Verification items for the finished model (mm, model axes). A direction names the side the tool comes from. Give positions to 0.01 mm unless a question says otherwise; leave off trailing zeros. Loops run counter-clockwise (first coordinate to the right, second up) from the corner with the lowest first, then second, coordinate; pieces in that order, holes last. Notation, with made-up numbers: M 24.5,71.25 L 68.5,71.25 A13 ccw 68.5,84.25 Z; hole C -4.5,58 d1. An arc over 180 degrees is marked long. Put each result on its own line as item: value. Start each with the question number.
from build123d import *

# Parameters (mm, degrees)
BOSS_EXTRUDE1_DEPTH = 79.7052
SKETCH5_R           = 5.499261314
SKETCH5_R_2         = 4.7625
CUT_EXTRUDE2_DEPTH  = 7.9375


with BuildPart() as part:
    # Sketch1 → Boss-Extrude1 (new body)
    with BuildSketch(Plane.XY):
        Polygon((2.806881074, 4.728984419), (-2.691980104, 4.795322525), (-5.498861178, 0.066338106), (-2.806881074, -4.728984419), (2.691980104, -4.795322525), (5.498861178, -0.066338106), align=None)
    extrude(amount=BOSS_EXTRUDE1_DEPTH)

    # Sketch5 → Cut-Extrude2 (cut)
    with BuildSketch(Plane.XY.offset(79.7052)):
        Circle(SKETCH5_R)
        Circle(SKETCH5_R_2, mode=Mode.SUBTRACT)
    extrude(amount=-CUT_EXTRUDE2_DEPTH, mode=Mode.SUBTRACT)


solid = part.part
Q1. Scan lines: L1, parallel to Y at x = -1.5, z = 31; L2, parallel to Y at x = 0.5, z = 4; L3, parallel to Z at x = 2.75, y = 4. Record each from-to range of solid material in increasing order.
Q2. Cross-section at A-A, the plane z = 15. Record the boundary of the cut face in (x, y).
Q3. Set-up check for faces 1 (the face through (-3.78, -2.9, 75.79)), 2 (the face through (-2.4, -4.3, 71.768)), 3 (the face through (2.5, -4.3, 71.768)), 4 (the face through (-2.34, 4.32, 71.768)): record each of +Z, -Z, +X, -X, +Y, -Y from which the full face is reachable in a straight line by a thin tool's end or side.
Q4. Go/stop test with flat-tipped pins: pin 1 (1 mm diameter, centred on x = -0.5, z = 51.5, fed in from +Y); pin 2 (0.7 mm diameter, centred on x = 5, y = 0.5, fed in from +Z); pin 3 (2 mm diameter, centred on x = 4, z = 61.5, fed in from -Y); pin 4 (3 mm diameter, centred on y = 2, z = 64.5, fed in from -X). Record where each tip stops, or that it passes through.
Q5. Cross-section at B-B, the plane y = -1.5. Record the boundary of the cut face in (x, z).
Q6. Cross-section at C-C, the plane y = 4. Record the boundary of the cut face in (x, z).
Ans:
1. L1: y = -4.74 to 4.78
1. L2: y = -4.77 to 4.76
1. L3: z = 0 to 71.77
2. outline: M -5.5,0.07 L -2.81,-4.73 L 2.69,-4.8 L 5.5,-0.07 L 2.81,4.73 L -2.69,4.8 Z
3. face 1: +Z
3. face 2: +Z, -X, -Y
3. face 3: +Z, +X, -Y
3. face 4: +Z, -X, +Y
4. pin 1: stops at y = 4.77
4. pin 2: stops at z = 79.71
4. pin 3: stops at y = -4.28
4. pin 4: stops at x = -5.24
5. outline: M -4.62,0 L 4.65,0 L 4.65,71.77 L 4.52,71.77 L 4.52,79.71 L -4.52,79.71 L -4.52,71.77 L -4.62,71.77 Z
6. outline: M -3.16,0 L 3.22,0 L 3.22,71.77 L 2.58,71.77 L 2.58,79.71 L -2.58,79.71 L -2.58,71.77 L -3.16,71.77 Z
